Could you check a few things on this model? Use its own coordinates, in mm. A direction names the side the tool comes from. Give positions to 0.01 mm unless a question says otherwise; leave off trailing zeros. Loops run counter-clockwise (first coordinate to the right, second up) from the corner with the lowest first, then second, coordinate; pieces in that order, holes last.
1. Imagine slicing it at C-C (z = 22). List the corners of the cut face in (x, y) for me.
2. Imagine slicing it at D-D (y = 0.95). Count the separate pieces of the cut face and the enclosed holes in it, plus the area to 3 significant figures.
3. I need wall thicknesses on line 1 along X through (y, z) = (0.7, -7); line 2 along X through (y, z) = (0.2, -38.5); line 3 along X through (y, z) = (0.3, -20). Which ranges of each line are inside material? Lowest first, please.
4. For P1, Ø0.8, axis at x = 18, y = 1, coming from the +Z side, with a flat end and sliding along its axis, tell me the tip position at first contact or that it passes through.
5. Thinking about a two-plate mould opening in X: for faces 3 (the cylindrical face through (38.133, 0.783, -42.672)), 4 (the cylindrical face through (-52.557, 0.783, -20.616)), 5 (the flat face through (-65.629, 0.783, 8.408)), 6 (the cylindrical face through (43.18, 0.78, -28.74)), which applies, +X half, -X half, draft (parallel to the pull), parting line (faces both ways), or undercut?
6. Imagine slicing it at B-B (x = -17). List the corners of the cut face in (y, z) for me, plus the area to 3 significant figures.
7. Imagine slicing it at A-A (x = 10). List the corners of the cut face in (y, z) for me, plus the area to 3 significant figures.
8. For faces 1 (the flat face through (-58.03, 0.78, -22.13)), 2 (the cylindrical face through (-41.134, 0.783, -2.021)), which set-ups out of +Z, -Z, +X, -X, +Y, -Y let a thin tool reach every point of the face, with its end or its side?
Autodesk Inventor part; units mm, degrees
ref_plane "YZ Plane" through (0, 0, 0) normal (1, 0, 0) x (0, 1, 0)
ref_plane "XZ Plane" through (0, 0, 0) normal (0, 1, 0) x (-1, 0, 0)
ref_plane "XY Plane" through (0, 0, 0) normal (0, 0, 1) x (1, 0, 0)
sketch "Sketch1" plane through (0, 0, 0) normal (0, 1, 0) x (-1, 0, 0)
  line L0 (-37.8542, 0.1524) -> (35.8058, 0.1524)
  line L1 (43.4258, -7.4676) -> (43.4258, -23.2918)
  line L2 (35.8058, -30.9118) -> (-37.8542, -30.9118)
  line L3 (-45.4742, -23.2918) -> (-45.4742, -7.4676)
  arc A0 (-37.8542, 0.1524) -> (-45.4742, -7.4676) centre (-37.8542, -7.4676) ccw
  arc A1 (-45.4742, -23.2918) -> (-37.8542, -30.9118) centre (-37.8542, -23.2918) ccw
  arc A2 (35.8058, -30.9118) -> (43.4258, -23.2918) centre (35.8058, -23.2918) ccw
  arc A3 (43.4258, -7.4676) -> (35.8058, 0.1524) centre (35.8058, -7.4676) ccw
  circle A4 centre (-72.8662, -0.3634) radius 2.3114
  circle A5 centre (-54.9057, -18.324) radius 2.3114
  circle A6 centre (-58.1742, 5.2324) radius 2.3114
  circle A7 centre (56.1258, 5.2324) radius 2.3114
  circle A8 centre (-32.7742, -37.2618) radius 2.3114
  circle A9 centre (30.7258, -37.2618) radius 2.3114
  circle A10 centre (52.8574, -18.324) radius 2.3114
  circle A11 centre (70.8179, -0.3634) radius 2.3114
  circle A12 centre (34.8968, 17.5971) radius 2.3114
  circle A13 centre (25.9166, 26.5773) radius 2.3114
  circle A14 centre (25.9166, 17.5971) radius 2.3114
  arc A15 (75.308, -4.8536) -> (73.078, 5.5707) centre (70.8179, -0.3634) ccw
  arc A16 (58.386, 11.1665) -> (56.1258, 11.5824) centre (56.1258, 5.2324) ccw
  arc A17 (30.4067, 31.0675) -> (19.5666, 26.5773) centre (25.9166, 26.5773) ccw
  arc A18 (30.7258, -43.6118) -> (30.9592, -43.6075) centre (30.7258, -37.2618) ccw
  arc A19 (-75.1264, 5.5707) -> (-77.3564, -4.8536) centre (-72.8662, -0.3634) ccw
  arc A20 (-32.7742, -43.6118) -> (-31.4271, -43.4673) centre (-32.7742, -37.2618) ccw
  arc A21 (-58.1742, 11.5824) -> (-60.4344, 11.1665) centre (-58.1742, 5.2324) ccw
  line L4 (-75.1264, 5.5707) -> (-60.4344, 11.1665)
  line L5 (-77.3564, -4.8536) -> (-42.3179, -39.8921)
  line L6 (-33.3376, -43.6118) -> (31.2893, -43.6118)
  line L7 (75.308, -4.8536) -> (40.2695, -39.8921)
  line L8 (58.386, 11.1665) -> (73.078, 5.5707)
  line L9 (19.5666, 26.5773) -> (19.5666, 24.2824)
  line L10 (30.4067, 31.0675) -> (46.172, 15.3021)
  line L11 (55.1523, 11.5824) -> (56.1258, 11.5824)
  line L12 (-58.1742, 11.5824) -> (6.8666, 11.5824)
  arc A22 (-42.3179, -39.8921) -> (-33.3376, -43.6118) centre (-33.3376, -30.9118) ccw
  arc A23 (31.2893, -43.6118) -> (40.2695, -39.8921) centre (31.2893, -30.9118) ccw
  arc A24 (46.172, 15.3021) -> (55.1523, 11.5824) centre (55.1523, 24.2824) ccw
  arc A25 (6.8666, 11.5824) -> (19.5666, 24.2824) centre (6.8666, 24.2824) ccw
  point P0 (0, 0)
  point P1 (43.4258, -30.9118)
  point P2 (43.4258, 0.1524)
  point P3 (-45.4742, -30.9118)
  point P4 (43.4258, -30.9118)
  dimension "d2" = 7.62
  dimension "d20" = 12.7
extrude "Extrusion1" add sketch "Sketch1" along normal blind 1.5875
properties part number "gusset-2-3.25-fulll-brace"
Derived:
1. outline: (-39.47, 0) - (-19.36, 0) - (-19.36, 1.59) - (-39.47, 1.59) - close
2. separate pieces: 1
2. enclosed holes: 12
2. area: 4,370 mm2
3. line 1: x = -73.16 to -43.41, 45.46 to 75.21
3. line 2: x = -41.66 to -32.68, -28.77 to 30.82, 34.73 to 43.71
3. line 3: x = -60.16 to -54.45, -51.27 to -43.43, 45.47 to 53.31, 56.5 to 62.21
4. P1: stops at z = 11.58
5. face 3: +X half
5. face 4: undercut
5. face 5: -X half
5. face 6: undercut
6. outline: (0, -43.61) - (1.59, -43.61) - (1.59, -30.91) - (0, -30.91) - close; (0, 0.15) - (1.59, 0.15) - (1.59, 16.63) - (0, 16.63) - close
6. area: 46.3 mm2
7. outline: (0, -43.61) - (1.59, -43.61) - (1.59, -30.91) - (0, -30.91) - close; (0, 0.15) - (1.59, 0.15) - (1.59, 11.58) - (0, 11.58) - close
7. area: 38.3 mm2
8. face 1: -Z, -X, +Y, -Y
8. face 2: +Y, -Y
